Input: part model. Units: mm. Frame: model coordinates. Face numbers are marked on the shaded views. A direction names the side the tool comes from. Round coordinates to 2 decimals unless told otherwise and drop trailing zeros. Loops run counter-clockwise (first coordinate to the right, second up) from the corner with the lowest first, then second, coordinate; pieces in that order, holes last. Notation, with made-up numbers: (28, 75) -> (83, 75) arc R18 cw to (83, 85) -> close; hole circle Ø8 at (-30, 8.5). An arc over 180 degrees is marked (long way). Answer as a JSON object with one key per item and string values.
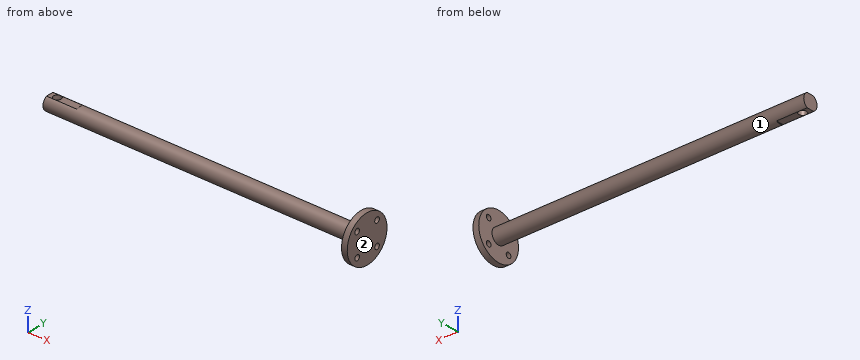
```python
from build123d import *

# Parameters (mm, degrees)
SKETCH1_R                       = 19.05
BOSS_EXTRUDE1_DEPTH             = 263.525
SKETCH2_W                       = 258.7625
SKETCH2_H                       = 12.7
CUT_EXTRUDE1_DEPTH              = 265.898528922
CUT_EXTRUDE1_DEPTH_BACK         = 265.898528922
SKETCH8_W                       = 25.4
SKETCH8_H                       = 0.79375
F_1_1_DIAMETER_HOLE2_D          = 6.35
F_16_0_177_DIAMETER_HOLE1_D     = 4.4958
F_16_0_177_DIAMETER_HOLE1_DEPTH = 25.4
F_16_0_177_DIAMETER_HOLE1_TIP   = 1.350674586


with BuildPart() as part:
    # Sketch1 → Boss-Extrude1 (new body)
    with BuildSketch(Plane(origin=(0, 0, 0), x_dir=(0, 0, -1), z_dir=(1, 0, 0))):
        Circle(SKETCH1_R)
    extrude(amount=BOSS_EXTRUDE1_DEPTH)

    # Sketch2 → Cut-Revolve1 (revolve, cut)
    with BuildSketch(Plane.XY, mode=Mode.PRIVATE) as cut_revolve1_sk:
        with Locations((129.38125, 12.7)):
            Rectangle(SKETCH2_W, SKETCH2_H)
    revolve(cut_revolve1_sk.sketch.rotate(Axis((-16.52066387, 0, 0), (1, 0, 0)), 90), axis=Axis((-16.52066387, 0, 0), (1, 0, 0)), mode=Mode.SUBTRACT)

    # Sketch8 → Cut-Extrude1 (cut, two sides: drawn at the far end of the back side and taken through both)
    with BuildSketch(Plane(origin=(0, 0, 0), x_dir=(1, 0, 0), z_dir=(0, 1, 0)).offset(-CUT_EXTRUDE1_DEPTH_BACK)):
        with Locations((12.7, 5.953125)):
            Rectangle(SKETCH8_W, SKETCH8_H)
        with Locations((12.7, -5.953125)):
            Rectangle(SKETCH8_W, SKETCH8_H)
    extrude(amount=CUT_EXTRUDE1_DEPTH + CUT_EXTRUDE1_DEPTH_BACK, mode=Mode.SUBTRACT)

    # 1 (1) Diameter Hole2 (through all)
    with Locations(Plane(origin=(0, 0, -5.55625), x_dir=(-1, 0, 0), z_dir=(0, 0, -1))):
        with Locations((-6.35, 0)):
            Hole(F_1_1_DIAMETER_HOLE2_D / 2)

    # #16 (0.177) Diameter Hole1
    with Locations(Plane.ZY.offset(-258.7625)):
        with Locations((9.525, 9.525), (-9.525, -9.525), (-9.525, 9.525), (9.525, -9.525)):
            Hole(F_16_0_177_DIAMETER_HOLE1_D / 2, depth=F_16_0_177_DIAMETER_HOLE1_DEPTH)
            with Locations((0, 0, -(F_16_0_177_DIAMETER_HOLE1_DEPTH + F_16_0_177_DIAMETER_HOLE1_TIP / 2))):  # 118° drill point
                Cone(0, F_16_0_177_DIAMETER_HOLE1_D / 2, F_16_0_177_DIAMETER_HOLE1_TIP, mode=Mode.SUBTRACT)


solid = part.part
```
1) Ray query, probe 1 along X at (y, z) = (-16.5, -9) (1 decimal); probe 2 along Y at (x, z) = (6, 3); probe 3 along Z at (x, y) = (182.5, -3). Return the intervals inside material, ascending.
Output:
{"probe 1": "x = 258.8 to 263.5", "probe 2": "y = -5.6 to -3.16, 3.16 to 5.6", "probe 3": "z = -5.6 to 5.6"}
2) Reachability of the marked faces 1 and 2 from +Z, -Z, +X, -X, +Y, -Y: full face, straight path, thin tool, end or side. Return the list, or none.
Output:
{"face 1": "-X", "face 2": "+Z, -Z, +X, +Y, -Y"}
3) Section C-C, the plane x = 37.5. Output: boundary loops of the cut face in (y, z), plus the area to 3 significant figures.
Output:
{"outline": "circle Ø12.7 at (0, 0)", "area": "127 mm^2"}
4) Section D-D, the plane z = 16. Output: boundary loops of the cut face in (x, y) (1 decimal), plus the area to 3 significant figures.
Output:
{"outline": "(258.8, -10.3) -> (263.5, -10.3) -> (263.5, 10.3) -> (258.8, 10.3) -> close", "area": "98.5 mm^2"}
5) Contact query for flat-ended pins moving along their axis: P1, Ø3, axis at x = 83.5, y = -3.5, coming from the -Z side; P2, Ø8.5, axis at x = 6.35, y = 0, coming from the +Z side; P3, Ø5, axis at y = -9.525, z = -9.525, coming from the +X side (3 decimals); P4, Ø0.6, axis at y = -1.5, z = 6, coming from the -X side. Output: stop coordinate, or through.
Output:
{"P1": "stops at z = -6.03", "P2": "stops at z = 5.56", "P3": "stops at x = 263.525", "P4": "stops at x = 25.4"}
